from build123d import *

# Parameters (mm, degrees)
F1_DEPTH = 6.35
F3_D     = 19.05
F5_DEPTH = 6.351


with BuildPart() as f1:
    # F0 (on Front) → F1 (new body)
    with BuildSketch(Plane.XZ):
        with BuildLine():
            ThreePointArc((76.2, 44.45), (72.480256, 53.430256), (63.5, 57.15))
            Line((63.5, 57.15), (-63.5, 57.15))
            ThreePointArc((-63.5, 57.15), (-72.480256, 53.430256), (-76.2, 44.45))
            Line((-76.2, 44.45), (-76.2, -44.45))
            ThreePointArc((-76.2, -44.45), (-72.480256, -53.430256), (-63.5, -57.15))
            Line((-63.5, -57.15), (63.5, -57.15))
            ThreePointArc((63.5, -57.15), (72.480256, -53.430256), (76.2, -44.45))
            Line((76.2, -44.45), (76.2, 44.45))
        make_face()
    extrude(amount=F1_DEPTH)

    # F3 (through all)
    with Locations(Plane.XZ.offset(6.35)):
        with Locations((38.1, 31.75), (38.1, 0), (38.1, -31.75)):
            Hole(F3_D / 2)

    # F4 (on face) → F5 (cut, through all)
    with BuildSketch(Plane.XZ.offset(6.35)):
        with BuildLine():
            Line((-12.7, 42.037003), (-63.5, 42.037003))
            ThreePointArc((-63.5, 42.037003), (-66.675, 38.862003), (-63.5, 35.687003))
            Line((-63.5, 35.687003), (-12.7, 35.687003))
            ThreePointArc((-12.7, 35.687003), (-9.525, 38.862003), (-12.7, 42.037003))
        make_face()
    extrude(amount=-F5_DEPTH, mode=Mode.SUBTRACT)


solid = f1.part
The listing builds one solid part. Answer for the finished solid, in the listing's coordinates (mm). A direction names the side the tool comes from. Coordinates: 2 decimals unless noted, no trailing zeros. Loops run counter-clockwise (first coordinate to the right, second up) from the corner with the lowest first, then second, coordinate; pieces in that order, holes last.
1) A tool of negligible diameter and unlimited length cuts with its end or side. For faces 4 (the face through (76.2, -3, -1)), 5 (the face through (-38, -3, 35.687)), from which of +Z, -Z, +X, -X, +Y, -Y can it reach the whole face along a straight path? Write none if from no direction.
2) Find section D-D on x = -19. Write down the section's boundary in (y, z), then the cut area to 3 significant figures.
3) Determine the mould class of faces 1 (the face through (72.58, -3.13, 53.33)), 2 (the face through (-72.58, -3.13, -53.33)), 3 (the face through (33.7, -3.1, -40.2)) for opening direction Z: pulls with the +Z half, pulls with the -Z half, needs draft (parallel to the pull), parting line crosses it, or undercut.
4) Flat-ended cylindrical pins translate along their axes: pin 1 Ø11.5 at (x, z) = (38.1, 31.75) entering from -Y; pin 2 Ø4 at (x, z) = (-54, 44.5) entering from +Y. Find the tip coordinate at first contact, or state that the pin passes through.
5) Find section C-C on z = 25.5. Write down the section's boundary in (x, y), then the cut area to 3 significant figures.
6) Find section B-B on y = -3.5. Write down the section's boundary in (x, z) (3 decimals).
7) Find section A-A on x = 38.1. Write down the section's boundary in (y, z) (3 decimals).
8) Find the intervals of material crossed by L1, parallel to Z at x = 38.1, y = -2 (3 decimals); L2, parallel to Z at x = -37, y = -3.25; L3, parallel to X at y = -3.5, z = -32, in increasing order.
Values:
1. face 4: +Z, -Z, +X, +Y, -Y
1. face 5: +Y, -Y
2. outline: (-6.35, -57.15) - (0, -57.15) - (0, 35.69) - (-6.35, 35.69) - close; (-6.35, 42.04) - (0, 42.04) - (0, 57.15) - (-6.35, 57.15) - close
2. area: 685 mm2
3. face 1: pulls with the +Z half
3. face 2: pulls with the -Z half
3. face 3: undercut
4. pin 1: passes through
4. pin 2: stops at y = 0
5. outline: (-76.2, -6.35) - (30.91, -6.35) - (30.91, 0) - (-76.2, 0) - close; (45.29, -6.35) - (76.2, -6.35) - (76.2, 0) - (45.29, 0) - close
5. area: 876 mm2
6. outline: (-76.2, -44.45) arc R12.7 ccw to (-63.5, -57.15) - (63.5, -57.15) arc R12.7 ccw to (76.2, -44.45) - (76.2, 44.45) arc R12.7 ccw to (63.5, 57.15) - (-63.5, 57.15) arc R12.7 ccw to (-76.2, 44.45) - close; hole (-63.5, 35.687) - (-12.7, 35.687) arc R3.175 ccw to (-12.7, 42.037) - (-63.5, 42.037) arc R3.175 ccw to start; hole circle Ø19.05 at (38.1, -31.75); hole circle Ø19.05 at (38.1, 0); hole circle Ø19.05 at (38.1, 31.75)
7. outline: (-6.35, -57.15) - (0, -57.15) - (0, -41.275) - (-6.35, -41.275) - close; (-6.35, -22.225) - (0, -22.225) - (0, -9.525) - (-6.35, -9.525) - close; (-6.35, 9.525) - (0, 9.525) - (0, 22.225) - (-6.35, 22.225) - close; (-6.35, 41.275) - (0, 41.275) - (0, 57.15) - (-6.35, 57.15) - close
8. L1: z = -57.15 to -41.275, -22.225 to -9.525, 9.525 to 22.225, 41.275 to 57.15
8. L2: z = -57.15 to 35.69, 42.04 to 57.15
8. L3: x = -76.2 to 28.58, 47.62 to 76.2
